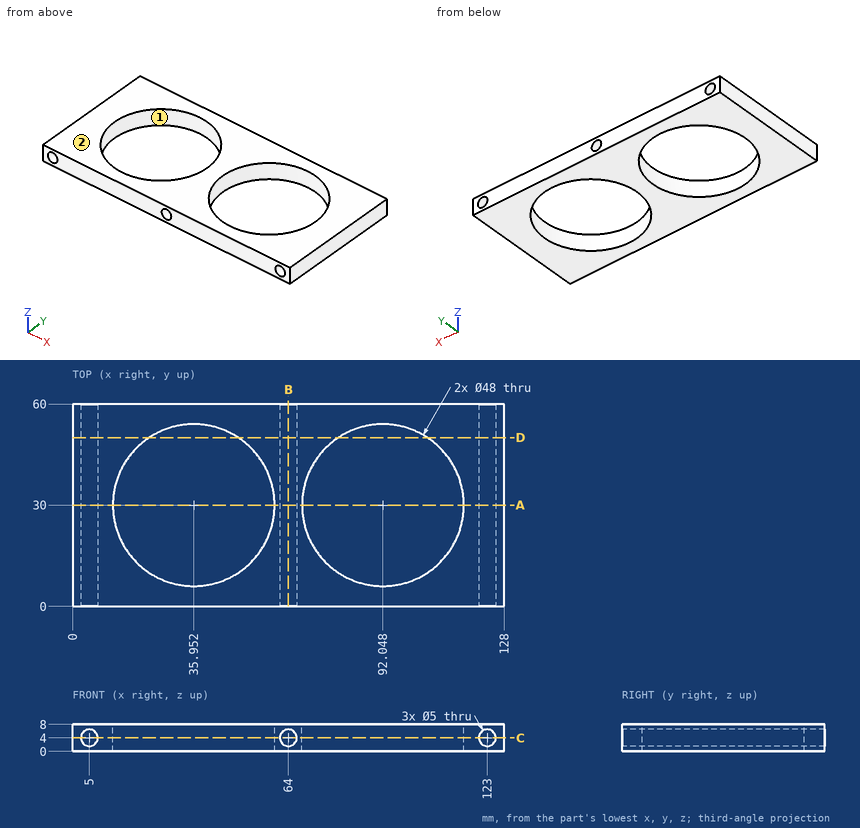
Verification items for this drawing (mm, ordinates from the low corner). Round coordinates to 2 decimals unless told otherwise and drop trailing zeros. Loops run counter-clockwise (first coordinate to the right, second up) from the corner with the lowest first, then second, coordinate; pieces in that order, holes last. Notation, with made-up numbers: (-18.75, 31.5) -> (14.25, 31.5) arc R20 cw to (14.25, 50.5) -> close; hole circle Ø1 at (38, 77.5). An arc over 180 degrees is marked (long way). Answer in a Markdown table with one row per item.
Q1. Thickness scan on L1, parallel to X at y = 29.5, z = 4; L2, parallel to X at y = 23, z = 4 (1 decimal); L3, parallel to Z at x = 5, y = 44. Record the ranges inside material, lowest first.
Data:
| item | result |
|---|---|
| L1 | x = 0 to 2.5, 7.5 to 11.96, 59.95 to 61.5, 66.5 to 68.05, 116.04 to 120.5, 125.5 to 128 |
| L2 | x = 0 to 2.5, 7.5 to 13, 58.9 to 61.5, 66.5 to 69.1, 115 to 120.5, 125.5 to 128 |
| L3 | z = 0 to 1.5, 6.5 to 8 |
Q2. Release check for a two-part mould opening along X. For the marked faces 1 and 2 record: released by +X, released by -X, zero draft, split by the parting line, or undercut.
Data:
| item | result |
|---|---|
| face 1 | undercut |
| face 2 | zero draft |
Q3. Sectioned sample at C-C on z = 4. Enter the section's corners in (x, y).
Data:
| item | result |
|---|---|
| outline | (0, 0) -> (2.5, 0) -> (2.5, 60) -> (0, 60) -> close; (7.5, 0) -> (61.5, 0) -> (61.5, 60) -> (7.5, 60) -> close; (66.5, 0) -> (120.5, 0) -> (120.5, 60) -> (66.5, 60) -> close; (125.5, 0) -> (128, 0) -> (128, 60) -> (125.5, 60) -> close; hole circle Ø48 at (35.95, 30); hole circle Ø48 at (92.05, 30) |
Q4. Go/stop test with flat-tipped pins: P1, Ø10, axis at x = 34, y = 48, coming from the -Z side; P2, Ø5, axis at x = 55.5, y = 41, coming from the +Z side. Record where each tip stops, or that it passes through.
Data:
| item | result |
|---|---|
| P1 | passes through |
| P2 | stops at z = 8 |
Q5. Sectioned sample at B-B on x = 64. Enter the section's corners in (y, z), then the cut area to 3 significant figures.
Data:
| item | result |
|---|---|
| outline | (0, 0) -> (60, 0) -> (60, 1.5) -> (0, 1.5) -> close; (0, 6.5) -> (60, 6.5) -> (60, 8) -> (0, 8) -> close |
| area | 180 mm^2 |
Q6. Sectioned sample at A-A on y = 30. Enter the section's corners in (x, z), then the cut area to 3 significant figures.
Data:
| item | result |
|---|---|
| outline | (0, 0) -> (11.95, 0) -> (11.95, 8) -> (0, 8) -> close; (59.95, 0) -> (68.05, 0) -> (68.05, 8) -> (59.95, 8) -> close; (116.05, 0) -> (128, 0) -> (128, 8) -> (116.05, 8) -> close; hole circle Ø5 at (5, 4); hole circle Ø5 at (64, 4); hole circle Ø5 at (123, 4) |
| area | 197 mm^2 |
Q7. Sectioned sample at D-D on y = 50. Enter the section's corners in (x, z) (1 decimal).
Data:
| item | result |
|---|---|
| outline | (0, 0) -> (22.7, 0) -> (22.7, 8) -> (0, 8) -> close; (49.2, 0) -> (78.8, 0) -> (78.8, 8) -> (49.2, 8) -> close; (105.3, 0) -> (128, 0) -> (128, 8) -> (105.3, 8) -> close; hole circle Ø5 at (5, 4); hole circle Ø5 at (64, 4); hole circle Ø5 at (123, 4) |
